The model under review builds one solid part; all positions refer to its coordinate system, in mm. Face numbers are marked on the shaded views. A direction names the side the tool comes from. Round coordinates to 2 decimals unless told otherwise and drop trailing zeros. Write each loop counter-clockwise with the first axis right and the second up, starting at its lowest first coordinate (ties: lowest second). Pieces come first, ordered by that corner, then holes. Notation, with made-up numbers: M 37.5,22.5 L 55.5,22.5 A6 ccw 55.5,33.5 Z; hole C 81.25,64.25 d8. An arc over 180 degrees is marked long. Write item = value, one per line. Start each with the question number.
Item 1: Tool access review of the marked faces 4, 5 and 6: name each direction out of +Z, -Z, +X, -X, +Y, -Y from which nothing blocks a thin tool from reaching the whole face with its end or side.
Item 2: For pin 1 Ø1 at (x, y) = (5, 11.5) entering from -Z; pin 2 Ø1.6 at (x, z) = (0, 0) entering from -Y; pin 3 Ø5 at (y, z) = (20.5, -1) entering from +X; pin 4 Ø1.5 at (x, z) = (0, 5) entering from +Y, all flat-tipped, find the tip position at first contact; note any pin that passes through.
Item 3: To check wall thickness, follow line 1 along X through (y, z) = (21.5, 0); line 2 along Z through (x, y) = (-0.75, 7.5); line 3 along Z through (x, y) = (-2.25, 2.75). State the ranges of each line that lie inside material, in increasing order.
Item 4: Take a section at A-A, the plane x = 0. Give the boundary of the cut face in (y, z) (3 decimals), plus the area to 3 significant figures.
Item 5: The part is to be moulded in two halves that separate along Z. For the marked faces 1, 2 and 3, say which applies: +Z half, -Z half, draft (parallel to the pull), parting line (faces both ways), or undercut.
Item 6: Take a section at B-B, the plane y = 18. Give the boundary of the cut face in (x, z), plus the area to 3 significant figures.
from build123d import *
from OCP.BRepFilletAPI import BRepFilletAPI_MakeChamfer

# Parameters (mm, degrees)
SKETCH2_R           = 1
BOSS_EXTRUDE1_DEPTH = 4
CHAMFER1_SIZE       = 0.5
CHAMFER1_SIZE2      = 0.555807111


with BuildPart() as part:
    # Sketch1 → Revolve1 (revolve)
    with BuildSketch(Plane.XY, mode=Mode.PRIVATE) as revolve1_sk:
        Polygon((1, 25), (2, 25), (2, 15), (7, 15), (5.55625, 0), (3.55625, 0), (3.55625, 12), (1, 12), align=None)
    revolve(revolve1_sk.sketch.rotate(Axis((0, 0, 0), (0, 1, 0)), 90), axis=Axis((0, 0, 0), (0, 1, 0)))

    # Sketch2 → Boss-Extrude1 (add)
    with BuildSketch(Plane(origin=(0, 15, 0), x_dir=(1, 0, 0), z_dir=(0, 1, 0))):
        Polygon((-8.248891971, 0), (-4.124445986, -7.14375), (4.124445986, -7.14375), (8.248891971, 0), (4.124445986, 7.14375), (-4.124445986, 7.14375), align=None)
        with Locations(Location((0, 0, 0), (0, 0, 90))):
            Circle(SKETCH2_R, mode=Mode.SUBTRACT)
    extrude(amount=-BOSS_EXTRUDE1_DEPTH)

    # Chamfer1: one chamfer whose edges measure the first distance from different faces: ONE call of the kernel's chamfer builder (chamfer() names one face for all edges)
    chamfer1_edges_1 = [part.edges().sort_by_distance(p)[0] for p in [
        (0, 0, 5.55625),
    ]]
    chamfer1_side_1 = [part.faces().sort_by_distance(p)[0] for p in [
        (0, 5.5, 6.085625),
    ]]
    chamfer1_edges_2 = [part.edges().sort_by_distance(p)[0] for p in [
        (0, 25, 2),
    ]]
    chamfer1 = BRepFilletAPI_MakeChamfer(part.part.solid().wrapped)
    for e in chamfer1_edges_1:
        chamfer1.Add(CHAMFER1_SIZE, CHAMFER1_SIZE2, e.wrapped, chamfer1_side_1[0].wrapped)  # the first distance lies on this face
    for e in chamfer1_edges_2:
        chamfer1.Add(CHAMFER1_SIZE, e.wrapped)
    add(Compound.cast(chamfer1.Shape()), mode=Mode.REPLACE)


solid = part.part
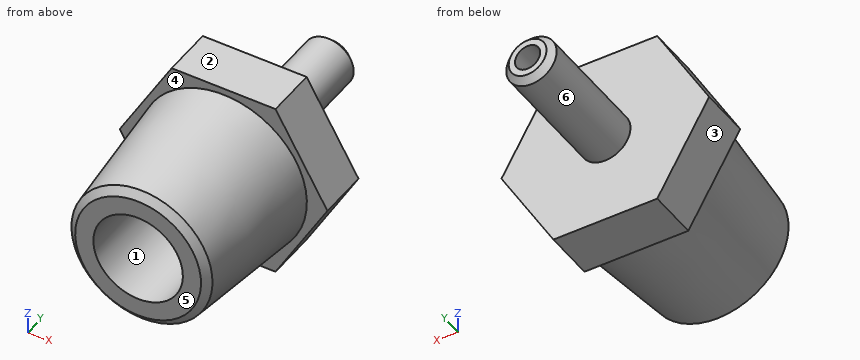
Response values:
q1.face_4 = -Y
q1.face_5 = +Z, -Z, +X, -X, -Y
q1.face_6 = +Y
q2.pin_1 = -6.49
q2.pin_2 = through
q2.pin_3 = 2
q2.pin_4 = 15
q3.line_1 = -2 to -1, 1 to 2
q3.line_2 = -6.23 to -3.48, 3.48 to 6.23
q3.line_3 = -5.37 to -2.75, 2.75 to 5.37
q4.outline = M 0,-5 L 0.498,-5.604 L 11,-6.615 L 11,-7.144 L 15,-7.144 L 15,-2 L 24.5,-2 L 25,-1.5 L 25,-1 L 11,-1 L 11,-3.556 L 0,-3.556 Z; M 0,3.556 L 11,3.556 L 11,1 L 25,1 L 25,1.5 L 24.5,2 L 15,2 L 15,7.144 L 11,7.144 L 11,6.615 L 0.498,5.604 L 0,5 Z
q4.area = 124 mm2
q5.face_1 = undercut
q5.face_2 = +Z half
q5.face_3 = -Z half
q6.outline = C 0,0 d4; hole C 0,0 d2
q6.area = 9.42 mm2
